Geometry check sheet. Reference: the model listing, model coordinates, mm. A direction names the side the tool comes from. Coordinates: 2 decimals unless noted, no trailing zeros. Write each loop counter-clockwise with the first axis right and the second up, starting at its lowest first coordinate (ties: lowest second). Pieces come first, ordered by that corner, then holes. Notation, with made-up numbers: M -22,46.25 L 29,46.25 A35 cw 29,79.25 Z; hole C 61.5,-22.75 d2. An arc over 180 degrees is marked long. Put each result on its own line as item: value. Start each with the question number.
1) Cross-section at B-B on x = 10.5. Record the cut outline in (y, z), plus the area to 3 significant figures.
2) Cross-section at C-C on x = 4. Record the cut outline in (y, z), plus the area to 3 significant figures.
3) Cross-section at D-D on z = 6. Record the cut outline in (x, y).
4) Cross-section at A-A on z = 3. Record the cut outline in (x, y).
5) Mould release check, pull along X, two halves, no side actions. Record for faces 6 (the conical face through (19.515, 5.787, 19.635)), 7 (the flat face through (0, 8, 9)), 8 (the flat face through (23, 7.3, 18)), 9 (the cylindrical face through (19.65, 5.82, 9.89)): released by +X, released by -X, zero draft, split by the parting line, or undercut.
6) Gauge pin test, flat ends, axial feed: pin 1 (2 mm diameter, centred on x = 6, y = 1.5, fed in from +Z); pin 2 (1 mm diameter, centred on x = 21, z = 10, fed in from +Y); pin 3 (1.4 mm diameter, centred on x = 22.5, y = 6, fed in from +Z). Record the tip position at first contact, or that the pin passes through.
7) Set-up check for faces 1 (the cylindrical face through (1.602, 1.556, 5.564)), 2 (the flat face through (23, 6, 16)), 3 (the flat face through (2, 3.157, 10)), 4 (the flat face through (4, 8, 19)), 5 (the cylindrical face through (11, 3.62, 10.14)): record each of +Z, -Z, +X, -X, +Y, -Y from which the full face is reachable in a straight line by a thin tool's end or side.
8) Scan lines: line 1 along X through (y, z) = (7.8, 10); line 2 along X through (y, z) = (3, 13); line 3 along Z through (x, y) = (4, 9.5). Record each from-to range of solid material in increasing order.
from build123d import *

# Parameters (mm, degrees)
F0_W      = 24
F0_H      = 11.5
F1_DEPTH  = 20
F2_R      = 3
F2_R_2    = 1.55
F3_DEPTH  = 20.001
F4_R      = 1.5
F4_R_2    = 1.4554355897
F4_R_3    = 1.5000002072
F5_DEPTH  = 11.501
F7_DEPTH  = 4
F9_DEPTH  = 1
F10_SIZE  = 0.5
F11_W     = 14.3343711684
F11_H     = 1.1
F12_DEPTH = 19.0010001


with BuildPart() as f1:
    # F0 (on Top) → F1 (new body)
    with BuildSketch(Plane.XY):
        with Locations((12, 5.75)):
            Rectangle(F0_W, F0_H)
    extrude(amount=F1_DEPTH)

    # F2 (on face) → F3 (cut, through all)
    with BuildSketch(Plane.XY.offset(20)):
        with Locations((8, 3.723813377)):
            Circle(F2_R)
        with Locations((15.5, 4.5)):
            Circle(F2_R)
        with Locations((21.2, 5.75)):
            Circle(F2_R_2)
    extrude(amount=-F3_DEPTH, mode=Mode.SUBTRACT)

    # F4 (on face) → F5 (cut, through all)
    with BuildSketch(Plane.XZ):
        with Locations((21.2, 10)):
            Circle(F4_R)
        with Locations((3.0564678513, 5.5)):
            Circle(F4_R_2)
        with Locations((3.1612319104, 15)):
            Circle(F4_R_3)
    extrude(amount=-F5_DEPTH, mode=Mode.SUBTRACT)

    # F6 (on face) → F7 (cut)
    with BuildSketch(Plane.XY.offset(20)):
        with BuildLine():
            Line((24, 7.3), (21.2, 7.3))
            ThreePointArc((21.2, 7.3), (22.2960155108, 6.8460155108), (22.75, 5.75))
            ThreePointArc((22.75, 5.75), (22.2960155108, 4.6539844892), (21.2, 4.2))
            Line((21.2, 4.2), (24, 4.2))
            Line((24, 4.2), (24, 7.3))
        make_face()
    extrude(amount=-F7_DEPTH, mode=Mode.SUBTRACT)

    # F8 (on face) → F9 (cut)
    with BuildSketch(Plane.XY.offset(20)):
        with BuildLine():
            Line((8, 6.723813377), (8, 11.5))
            Line((8, 11.5), (0, 11.5))
            Line((0, 11.5), (0, 0))
            Line((0, 0), (8, 0))
            Line((8, 0), (8, 0.723813377))
            ThreePointArc((8, 0.723813377), (5, 3.723813377), (8, 6.723813377))
        make_face()
    extrude(amount=-F9_DEPTH, mode=Mode.SUBTRACT)

    # F10
    f10_edges = [f1.edges().sort_by_distance(p)[0] for p in [
        (4, 0, 19),
        (0, 5.75, 19),
        (0, 0, 9.5),
        (0, 11.5, 9.5),
        (8, 9.111907, 20),
        (8, 0.361907, 20),
        (8, 0, 19.5),
        (16, 0, 20),
        (24, 2.1, 20),
        (22.6, 4.2, 20),
        (24, 9.4, 20),
        (16, 11.5, 20),
        (24, 0, 10),
        (0, 5.75, 0),
        (12, 0, 0),
        (24, 5.75, 0),
        (12, 11.5, 0),
        (24, 11.5, 10),
        (4, 11.5, 19),
        (8, 11.5, 19.5),
        (12.5, 4.5, 20),
    ]]
    chamfer(f10_edges, length=F10_SIZE)

    # F11 (on face) → F12 (cut, through all)
    with BuildSketch(Plane.XY.offset(19)):
        with Locations((3.4663419938, 3.7068520686)):
            Rectangle(F11_W, F11_H)
    extrude(amount=-F12_DEPTH, mode=Mode.SUBTRACT)


solid = f1.part
Answer key:
1. outline: M 0,0.5 L 0.5,0 L 2.07,0 L 2.07,20 L 0.5,20 L 0,19.5 Z; M 5.38,0 L 11,0 L 11.5,0.5 L 11.5,19.5 L 11,20 L 5.38,20 Z
1. area: 163 mm²
2. outline: M 0,0.5 L 0.5,0 L 3.16,0 L 3.16,4.39 L 0,4.39 Z; M 0,6.61 L 3.16,6.61 L 3.16,13.76 L 0,13.76 Z; M 0,16.24 L 3.16,16.24 L 3.16,19 L 0.5,19 L 0,18.5 Z; M 4.26,0 L 11,0 L 11.5,0.5 L 11.5,4.39 L 4.26,4.39 Z; M 4.26,6.61 L 11.5,6.61 L 11.5,13.76 L 4.26,13.76 Z; M 4.26,16.24 L 11.5,16.24 L 11.5,18.5 L 11,19 L 4.26,19 Z
2. area: 148 mm²
3. outline: M 0,0.5 L 0.5,0 L 1.69,0 L 1.69,3.16 L 0,3.16 Z; M 0,4.26 L 1.69,4.26 L 1.69,11.5 L 0.5,11.5 L 0,11 Z; M 4.42,0 L 23.5,0 L 24,0.5 L 24,11 L 23.5,11.5 L 4.42,11.5 L 4.42,4.26 L 5.05,4.26 A3 cw long 5.05,3.16 L 4.42,3.16 Z; hole C 15.5,4.5 d6; hole C 21.2,5.75 d3.1
4. outline: M 0,0.5 L 0.5,0 L 23.5,0 L 24,0.5 L 24,11 L 23.5,11.5 L 0.5,11.5 L 0,11 L 0,4.26 L 5.05,4.26 A3 cw long 5.05,3.16 L 0,3.16 Z; hole C 15.5,4.5 d6; hole C 21.2,5.75 d3.1
5. face 6: released by +X
5. face 7: released by -X
5. face 8: zero draft
5. face 9: undercut
6. pin 1: stops at z = 19
6. pin 2: passes through
6. pin 3: stops at z = 16
7. face 1: +Y, -Y
7. face 2: +Z, +X
7. face 3: +Z, -Z, -X
7. face 4: +Z, -X, +Y, -Y
7. face 5: +Z, -Z
8. line 1: x = 0 to 19.7, 22.7 to 24
8. line 2: x = 0 to 5.09, 10.91 to 12.9, 18.1 to 24
8. line 3: z = 0 to 4.39, 6.61 to 13.76, 16.24 to 19
